Here's how the part is built. I have some questions about the finished solid (model axes, mm). Coordinates: 2 decimals unless noted, no trailing zeros. Loops run counter-clockwise (first coordinate to the right, second up) from the corner with the lowest first, then second, coordinate; pieces in that order, holes last. Notation, with made-up numbers: (0, 15.5) -> (5, 15.5) arc R17 cw to (5, 45.5) -> close; hole circle Ø3 at (80, 73.25). An arc over 180 degrees is marked (long way). Answer as a JSON object with one key per item and string values. Group by question number.
1) I need wall thicknesses on probe 1 along Y at (x, z) = (0, 3.75) (3 decimals); probe 2 along Z at (x, y) = (46.5, 3); probe 3 along X at (y, z) = (-9, 1.25). Which ranges of each line are inside material? Lowest first, please. Write a range as [from, to].
2) I want a section at B-B (x = 65). Write out the boundary of the cut face in (y, z).
3) I want a section at C-C (z = 1.75). Count the separate pieces of the cut face and the enclosed holes in it, then the cut area to 3 significant figures.
4) I'm going to push flat-ended pins straight in: pin 1 (4.5 mm diameter, centred on x = 8.24, y = 8.24, fed in from +Z); pin 2 (10 mm diameter, centred on x = 31.5, y = -7.5, fed in from -Z); pin 3 (4 mm diameter, centred on x = 63, z = 3, fed in from -Y); pin 4 (1.5 mm diameter, centred on y = 22.5, z = 2, fed in from -X). Where does each tip first touch, or does it pass through?
5) I want a section at D-D (x = 47.5). Write out the boundary of the cut face in (y, z), then the cut area to 3 significant figures.
```python
from build123d import *
from build123d.topology import SkipClean

# Parameters (mm, degrees)
SKETCH1_R             = 3.175
BOSS_EXTRUDE1_DEPTH   = 6.35
F_6_32_TAPPED_HOLE1_D = 2.7051
BOSS_EXTRUDE3_START   = 1.5875
SKETCH5_R             = 7
SKETCH5_R_2           = 3.175
BOSS_EXTRUDE3_DEPTH   = 1.5875


with BuildPart() as part:
    # Sketch1 → Boss-Extrude1 (new body)
    with BuildSketch(Plane.XY):
        with BuildLine():
            Line((0, -15.875), (12.7, -15.875))
            ThreePointArc((12.7, -15.875), (14.017406742, -15.736838655), (15.277486023, -15.328366764))
            ThreePointArc((15.277486023, -15.328366764), (44.45, -9.14146), (73.622513977, -15.328366764))
            ThreePointArc((73.622513977, -15.328366764), (79.912012711, -14.677034708), (82.52084196, -8.917170323))
            ThreePointArc((82.52084196, -8.917170323), (69.763837113, 21.925102015), (41.955075464, 40.382071192))
            ThreePointArc((41.955075464, 40.382071192), (39.851813107, 40.009159666), (38.89375, 38.1))
            add(Edge.make_bspline(
                [(38.89375, 38.1), (38.89375, 8.240619939), (68.342560944, 15.875), (0, 15.875)],
                knots=[0, 0, 0, 0, 1, 1, 1, 1], degree=3))
            ThreePointArc((0, 15.875), (-15.875, 0), (0, -15.875))
        make_face()
        Circle(SKETCH1_R, mode=Mode.SUBTRACT)
    extrude(amount=BOSS_EXTRUDE1_DEPTH)

    # #6-32 Tapped Hole1 (through all)
    with Locations(Plane.XY.offset(6.35)):
        with Locations((8.242390195, 8.242390195), (-8.242390195, 8.242390195), (8.242390195, -8.242390195), (-8.242390195, -8.242390195)):
            Hole(F_6_32_TAPPED_HOLE1_D / 2)

    # Sketch5 → Boss-Extrude3 (add)
    with SkipClean():  # the faces are left unmerged after this step: merging them gives an invalid solid
        with BuildSketch(Plane(origin=(0, 0, 0), x_dir=(-1, 0, 0), z_dir=(0, 0, -1)).offset(BOSS_EXTRUDE3_START)):
            Circle(SKETCH5_R)
            Circle(SKETCH5_R_2, mode=Mode.SUBTRACT)
        extrude(amount=-BOSS_EXTRUDE3_DEPTH)


solid = part.part
```
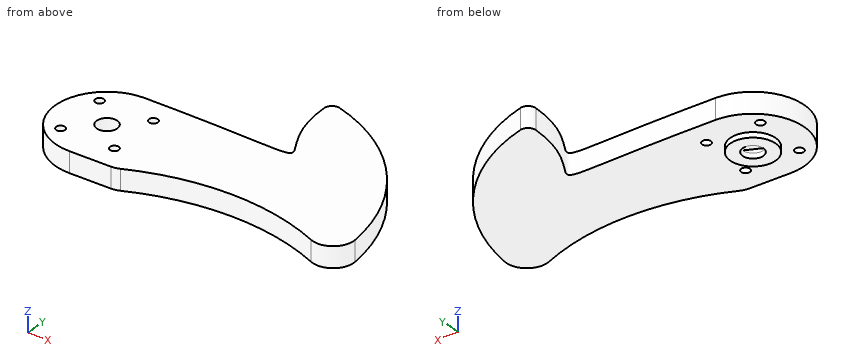
Determined:
{
 "1": {"probe 1": "[-15.875, -3.175], [3.175, 15.875]", "probe 2": "[0, 6.35]", "probe 3": "[-13.08, -9.36], [-7.12, 7.12], [9.36, 82.53]"},
 "2": {"outline": "(-12.14, 0) -> (27.04, 0) -> (27.04, 6.35) -> (-12.14, 6.35) -> close"},
 "3": {"separate pieces": "1", "enclosed holes": "5", "area": "3,100 mm^2"},
 "4": {"pin 1": "z = 6.35", "pin 2": "z = 0", "pin 3": "y = -12.14", "pin 4": "x = 41.86"},
 "5": {"outline": "(-9.21, 0) -> (38.41, 0) -> (38.41, 6.35) -> (-9.21, 6.35) -> close", "area": "302 mm^2"}
}
